CAD build for the part. Positions are in the model's coordinates, mm. A direction names the side the tool comes from. Give positions to 0.01 mm unless a question says otherwise; leave off trailing zeros. Order: outer loops, then holes, each group sorted by start corner. A loop starts at its lowest first (then second) coordinate and runs counter-clockwise, first axis right, second up. Notation, with made-up numbers: (-1.75, -29.75) -> (33.25, -29.75) arc R25 cw to (33.25, -1.75) -> close; hole circle Ø6 at (49.5, -38). An arc over 180 degrees is marked (long way). Answer as CSV lines item,"result".
```python
from build123d import *

# Parameters (mm, degrees)
CHAMFER_988_SIZE          = 1
SKETCH_2_W                = 4.1
SKETCH_2_H                = 2.45
PATTERN_LINEAR_O_2_COUNT  = 2
PATTERN_LINEAR_O_2_PITCH  = 9
SKETCH_3_W                = 2.4
SKETCH_3_H                = 4.1
PATTERN_CIRCULAR_M4_COUNT = 6


with BuildPart() as part:
    # Sketch 1 → Revolve 949 (revolve)
    with BuildSketch(Plane.XY, mode=Mode.PRIVATE) as revolve_949_sk:
        Polygon((-12, 40), (-12, 79), (0, 79), (0, 70.95), (25, 70.95), (25, 62), (0, 62), (0, 40), align=None)
    revolve(revolve_949_sk.sketch.rotate(Axis((0, 0, 0), (1, 0, 0)), 90), axis=Axis((0, 0, 0), (1, 0, 0)))

    # Chamfer 988
    chamfer_988_edges = [part.edges().sort_by_distance(p)[0] for p in [
        (25, 0, -70.95),
    ]]
    chamfer(chamfer_988_edges, length=CHAMFER_988_SIZE)

    # Sketch 2 → O_ G-135 (revolve, cut)
    with BuildSketch(Plane.XY, mode=Mode.PRIVATE) as o_g_135_sk:
        with Locations((7.05, 69.725)):
            Rectangle(SKETCH_2_W, SKETCH_2_H)
    o_g_135 = revolve(o_g_135_sk.sketch.rotate(Axis((0, 0, 0), (1, 0, 0)), 90), axis=Axis((0, 0, 0), (1, 0, 0)), mode=Mode.SUBTRACT)

    # Pattern Linear O_ 2: O_ G-135 ×2
    with Locations(*[(i * PATTERN_LINEAR_O_2_PITCH, 0, 0) for i in range(1, PATTERN_LINEAR_O_2_COUNT)]):
        add(o_g_135, mode=Mode.SUBTRACT)

    # Sketch 3 → O_ G-85 (revolve, cut)
    with BuildSketch(Plane.XY, mode=Mode.PRIVATE) as o_g_85_sk:
        with Locations((-10.8, 44.55)):
            Rectangle(SKETCH_3_W, SKETCH_3_H)
    revolve(o_g_85_sk.sketch.rotate(Axis((0, 0, 0), (1, 0, 0)), 90), axis=Axis((0, 0, 0), (1, 0, 0)), mode=Mode.SUBTRACT)

    # Sketch 4 → Hole Wizard M4 (revolve, cut)
    with BuildSketch(Plane(origin=(-12, 54.25, 0), x_dir=(0, 0, 1), z_dir=(0, 1, 0))):
        Polygon((0, 0), (0, 10.991420021), (1.65, 10), (1.65, 0), align=None)
    hole_wizard_m4 = revolve(axis=Axis((-18.35, 54.25, 0), (1, 0, 0)), mode=Mode.SUBTRACT)

    # Pattern Circular M4: Hole Wizard M4 ×6 about axis
    pattern_circular_m4_axis = Axis((0, 0, 0), (1, 0, 0))
    for i in range(1, PATTERN_CIRCULAR_M4_COUNT):
        add(hole_wizard_m4.rotate(pattern_circular_m4_axis, i * 360 / PATTERN_CIRCULAR_M4_COUNT), mode=Mode.SUBTRACT)


solid = part.part
```
1) Wall check: line 1 along Y through (x, z) = (-10, 0); line 2 along Y through (x, z) = (-10, -35.5); line 3 along X through (y, z) = (10, 43). Give the ranges that are in metal, low to high. Write a range as [from, to].
Data:
line 1,"y = [-79, -55.9], [-52.6, -46.6], [-42.5, -40], [40, 42.5], [46.6, 52.6], [55.9, 79]"
line 2,"y = [-70.57, -30.19], [-23.37, -18.43], [18.43, 23.37], [30.19, 70.57]"
line 3,"x = [-9.6, 0]"
2) Which spindle directions (+Z, -Z, +X, -X, +Y, -Y) get a long thin tool onto all of the face, cutting with end or side? Do faces 4 (the cylindrical face through (11.584, -47.951, -52.293)), 5 (the cylindrical face through (-10.783, -12.766, 40.537)), 6 (the flat face through (5, -58, 37)). Say none if no direction does.
Data:
face 4,"+X"
face 5,"-X"
face 6,"none"
3) Pin check, flat tips, straight feed: P1, Ø2, axis at y = 59.5, z = -5.5, coming from the +X side; P2, Ø6, axis at x = 7, z = -20.5, coming from the -Y side; P3, Ø2, axis at y = 54.25, z = 0, coming from the -X side. Stop position of each tip, or through.
Data:
P1,"stops at x = 0"
P2,"stops at y = -68.56"
P3,"stops at x = -1.61"
4) Pull direction Y, two halves, no side cores. Call faces 1 (the cylindrical face through (7.079, -20.576, 65.337)), 2 (the flat face through (0, -30, -65)), 3 (the cylindrical face through (12.325, -61.472, -8.071)): pulls with the +Y half, pulls with the -Y half, needs draft (parallel to the pull), parting line crosses it, or undercut.
Data:
face 1,"parting line crosses it"
face 2,"needs draft"
face 3,"undercut"
5) Band-saw the part on A-A, the plane x = -6. Write the cut outline in (y, z) (3 decimals), then the cut area to 3 significant figures.
Data:
outline,"circle Ø158 at (0, 0); hole circle Ø3.3 at (-54.25, 0); hole circle Ø80 at (0, 0); hole circle Ø3.3 at (-27.125, -46.982); hole circle Ø3.3 at (-27.125, 46.982); hole circle Ø3.3 at (27.125, -46.982); hole circle Ø3.3 at (27.125, 46.982); hole circle Ø3.3 at (54.25, 0)"
area,"14,500 mm2"
